Could you check a few things on this model? Use its own coordinates, in mm. Give positions to 0.01 mm unless a question says otherwise; leave off trailing zeros. Loops run counter-clockwise (first coordinate to the right, second up) from the corner with the lowest first, then second, coordinate; pieces in that order, holes last. Notation, with made-up numbers: (-8.75, 5) - (47.25, 5) arc R19 cw to (47.25, 15) - close; hole circle Ø7 at (82.25, -8). An arc over 180 degrees is marked (long way). Write each question's results on one line, items separated by ' | '. Start each with the question number.
```python
from build123d import *

# Parameters (mm, degrees)
SKETCH1_W           = 152.4
SKETCH1_H           = 177.8
BOSS_EXTRUDE1_DEPTH = 2.54
SKETCH2_R           = 19.05
CUT_EXTRUDE1_DEPTH  = 235.190203894
SKETCH3_R           = 6.35
CUT_EXTRUDE3_DEPTH  = 235.190203894


with BuildPart() as part:
    # Sketch1 → Boss-Extrude1 (new body)
    with BuildSketch(Plane.XY):
        with Locations((76.2, 88.9)):
            Rectangle(SKETCH1_W, SKETCH1_H)
    extrude(amount=BOSS_EXTRUDE1_DEPTH)

    # Sketch2 → Cut-Extrude1 (cut, through all)
    with BuildSketch(Plane.XY):
        with Locations((76.2, 88.9)):
            Circle(SKETCH2_R)
    extrude(amount=CUT_EXTRUDE1_DEPTH, mode=Mode.SUBTRACT)

    # Sketch3 → Cut-Extrude3 (cut, through all)
    with BuildSketch(Plane.XY):
        with Locations((19.05, 160.401)):
            Circle(SKETCH3_R)
        with Locations(Location((133.35, 160.401, 0), (0, 0, 180))):
            Circle(SKETCH3_R)
        with Locations((133.35, 17.399)):
            Circle(SKETCH3_R)
        with Locations(Location((19.05, 17.399, 0), (0, 0, 180))):
            Circle(SKETCH3_R)
    extrude(amount=CUT_EXTRUDE3_DEPTH, mode=Mode.SUBTRACT)


solid = part.part
```
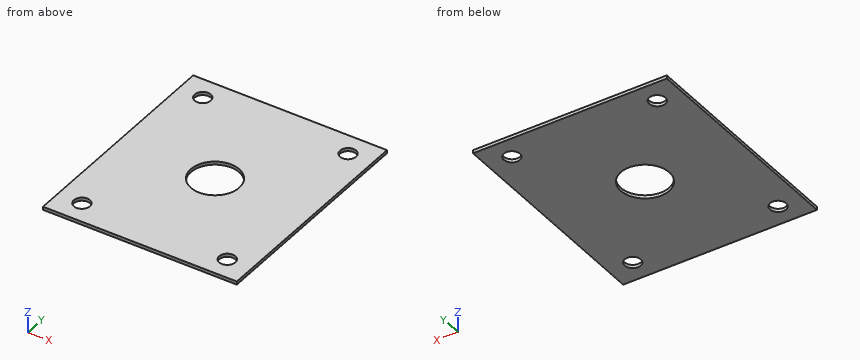
Q1. I want a section at A-A, the plane x = 133.35. List the corners of the cut face in (y, z) for me, then the cut area to 3 significant figures.
Q2. I want a section at D-D, the plane z = 1.5. List the corners of the cut face in (x, y) for me.
Q3. I need wall thicknesses on L1, parallel to Y at x = 133.35, z = 1; L2, parallel to Y at x = 134, z = 1.3; L3, parallel to X at y = 20, z = 1.9. Which ranges of each line are inside material? Lowest first, please. Write a range as from..to.
Q4. I want a section at B-B, the plane y = 88.9. List the corners of the cut face in (x, z) for me, then the cut area to 3 significant figures.
Q5. I want a section at C-C, the plane x = 76.2. List the corners of the cut face in (y, z) for me.
Conclusion:
1) outline: (0, 0) - (11.05, 0) - (11.05, 2.54) - (0, 2.54) - close; (23.75, 0) - (154.05, 0) - (154.05, 2.54) - (23.75, 2.54) - close; (166.75, 0) - (177.8, 0) - (177.8, 2.54) - (166.75, 2.54) - close | area: 387 mm^2
2) outline: (0, 0) - (152.4, 0) - (152.4, 177.8) - (0, 177.8) - close; hole circle Ø12.7 at (19.05, 17.4); hole circle Ø12.7 at (19.05, 160.4); hole circle Ø38.1 at (76.2, 88.9); hole circle Ø12.7 at (133.35, 17.4); hole circle Ø12.7 at (133.35, 160.4)
3) L1: 0..11.05, 23.75..154.05, 166.75..177.8 | L2: 0..11.08, 23.72..154.08, 166.72..177.8 | L3: 0..13.26, 24.84..127.56, 139.14..152.4
4) outline: (0, 0) - (57.15, 0) - (57.15, 2.54) - (0, 2.54) - close; (95.25, 0) - (152.4, 0) - (152.4, 2.54) - (95.25, 2.54) - close | area: 290 mm^2
5) outline: (0, 0) - (69.85, 0) - (69.85, 2.54) - (0, 2.54) - close; (107.95, 0) - (177.8, 0) - (177.8, 2.54) - (107.95, 2.54) - close
